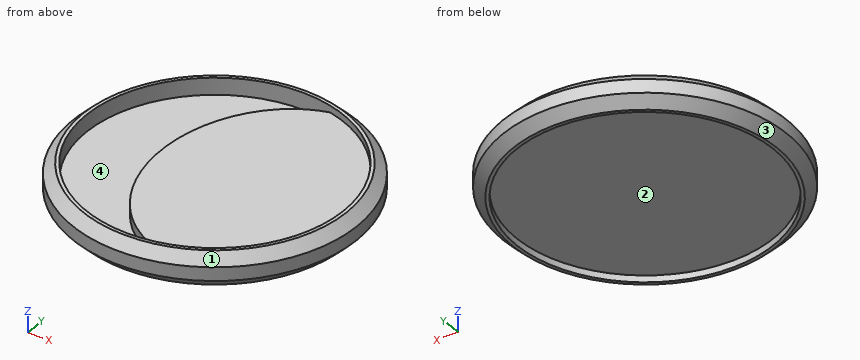
```python
from build123d import *

# Parameters (mm, degrees)
F0_R          = 10
F1_DEPTH      = 1.5
F3_DEPTH      = 0.75
F4_R          = 10.5
F4_R_2        = 9.5
F5_DEPTH      = 2
F5_DEPTH_BACK = 0.5
F6_SIZE       = 0.75


# Not quite as in the source:
# - a feature of the source that left no trace in its solid (it failed there, or was rolled back) is left out


with BuildPart() as f1:
    # F0 (on Top) → F1 (new body)
    with BuildSketch(Plane.XY):
        Circle(F0_R)
    extrude(amount=F1_DEPTH)

    # F2 (on face) → F3 (cut)
    with BuildSketch(Plane.XY.offset(1.5)):
        with BuildLine():
            add(Edge.make_bspline(
                [(3.2873270655, 9.444230025), (-3.9457486769, 8.7871247234), (-3.9457486769, 0), (-3.9457486769, -8.7871247234), (3.2873270655, -9.444230025)],
                knots=[0.0748503411, 0.0748503411, 0.0748503411, 1.5707963268, 1.5707963268, 3.0667423125, 3.0667423125, 3.0667423125], degree=2, weights=[1, 0.7330690514, 1, 0.7330690514, 1]))
            ThreePointArc((3.2873270655, 9.444230025), (-10, 0), (3.2873270655, -9.444230025))
        make_face()
    extrude(amount=-F3_DEPTH, mode=Mode.SUBTRACT)

    # F4 (on Top) → F5 (join, two sides)
    with BuildSketch(Plane.XY) as f5_sk:
        Circle(F4_R)
        Circle(F4_R_2, mode=Mode.SUBTRACT)
    extrude(amount=F5_DEPTH)
    extrude(f5_sk.sketch, amount=-F5_DEPTH_BACK)

    # F6
    f6_edges = [f1.edges().sort_by_distance(p)[0] for p in [
        (-10.5, 0, 2),
        (-10.5, 0, -0.5),
    ]]
    chamfer(f6_edges, length=F6_SIZE)


solid = f1.part
```
Could you check a few things on this model? Use its own coordinates, in mm. Face numbers are marked on the shaded views. A direction names the side the tool comes from. Coordinates: 2 decimals unless noted, no trailing zeros. Order: outer loops, then holes, each group sorted by start corner. A loop starts at its lowest first (then second) coordinate and runs counter-clockwise, first axis right, second up. Notation, with made-up numbers: M -23,-14 L 10,-14 A18 cw 10,16 Z; hole C -33,81 d4. An arc over 180 degrees is marked long. Use a Markdown table: item, result. Add a question column.
Q1. We'd pull the mould along X, two halves only. Please class the marked faces 1 and 2: pulls with the +X half, pulls with the -X half, needs draft (parallel to the pull), parting line crosses it, or undercut.
Q2. If I drill on L1, parallel to Y at x = 0, z = 0.95; L2, parallel to Y at x = -5.75, z = -0.1; L3, parallel to Z at x = 3, y = -7.25, over which ranges is the centre line in solid material (lowest first)?
Q3. Which directions (+Z, -Z, +X, -X, +Y, -Y) give clear straight access to the entire face, cutting with the end or side of a thin tool? Please do the marked faces 3 and 4.
Q4. I'm going to push flat-ended pins straight in: pin 1 (5 mm diameter, centred on x = -2.5, y = -2, fed in from -Z); pin 2 (9.5 mm diameter, centred on x = -1.5, y = 4, fed in from +Z); pin 3 (1.5 mm diameter, centred on y = -2.5, z = 1, fed in from -X). Where does each tip first touch, or does it pass through?
Q5. I want a section at A-A on z = 0.5. List the corners of the cut face in (x, y) for me, then the cut area to 3 significant figures.
Checked values:
| question | item | result |
|---|---|---|
| 1 | face 1 | parting line crosses it |
| 1 | face 2 | undercut |
| 2 | L1 | -10.5 to -9.5, -8.23 to 8.23, 9.5 to 10.5 |
| 2 | L2 | -8.36 to -7.56, 7.56 to 8.36 |
| 2 | L3 | 0 to 1.5 |
| 3 | face 3 | -Z |
| 3 | face 4 | +Z |
| 4 | pin 1 | z = 0 |
| 4 | pin 2 | z = 1.5 |
| 4 | pin 3 | x = -10.35 |
| 5 | outline | C 0,0 d21 |
| 5 | area | 346 mm² |
